For this review, take the finished solid that the model builds, in its own axes (mm). A direction names the side the tool comes from. Coordinates: 2 decimals unless noted, no trailing zeros. Write each loop counter-clockwise with the first axis right and the second up, starting at its lowest first coordinate (ties: lowest second). Pieces come first, ordered by that corner, then holes. Notation, with made-up numbers: (31.25, 74) - (49.25, 74) arc R23 ccw to (49.25, 100) - close; hole circle Ø3 at (58.25, -3.5). An arc over 180 degrees is marked (long way). Write each question's results on one line, items separated by ' | '.
from build123d import *

# Parameters (mm, degrees)
F0_W      = 140
F0_H      = 154
F1_DEPTH  = 54
F2_R      = 16
F3_DEPTH  = 140.001
F5_DEPTH  = 140.001
F6_W      = 25
F6_H      = 58
F7_DEPTH  = 46
F8_R      = 5
F9_ANGLE  = 270
F14_R     = 8
F15_DEPTH = 45
F16_R     = 5
F17_DEPTH = 120.001
F18_R     = 3
F19_DEPTH = 108.001


with BuildPart() as f1:
    # F0 (on Front) → F1 (new body, symmetric)
    with BuildSketch(Plane.XZ):
        with Locations((70, 0)):
            Rectangle(F0_W, F0_H)
    extrude(amount=F1_DEPTH, both=True)

    # F2 (on face) → F3 (cut, through all)
    with BuildSketch(Plane(origin=(0, 0, 0), x_dir=(0, -1, 0), z_dir=(-1, 0, 0))):
        with Locations((0, 48)):
            Circle(F2_R)
        with Locations((0, 3)):
            Circle(F2_R)
    extrude(amount=-F3_DEPTH, mode=Mode.SUBTRACT)

    # F4 (on face) → F5 (cut, through all)
    with BuildSketch(Plane(origin=(0, 0, 0), x_dir=(0, -1, 0), z_dir=(-1, 0, 0))):
        Polygon((-54, 77), (-54, 43), (-29, 43), (-29, 59.7311109304), (-11.6953058452, 77.0358050852), align=None)
        Polygon((54, 77), (11.6953058452, 77.0358050852), (29, 59.7311109304), (29, 43), (54, 43), align=None)
    extrude(amount=-F5_DEPTH, mode=Mode.SUBTRACT)

    # F6 (on face) → F7 (cut)
    with BuildSketch(Plane.XY.offset(77)):
        with Locations((127.5, 0)):
            Rectangle(F6_W, F6_H)
    extrude(amount=-F7_DEPTH, mode=Mode.SUBTRACT)

    # F8
    f8_edges = [f1.edges().sort_by_distance(p)[0] for p in [
        (127.5, -29, 31),
        (127.5, 29, 31),
    ]]
    fillet(f8_edges, radius=F8_R)


with BuildPart() as f1_1:
    # F9: moved
    add(f1.part.rotate(Axis((0, 0, -77), (0, 1, 0)), F9_ANGLE))


with BuildPart() as f1_2:
    # F11: moved
    add(f1_1.part.moved(Location((154, 0, 0))))


with BuildPart() as f1_3:
    # F13: moved
    add(f1_2.part.moved(Location((0, 0, 7))))

    # F14 (on face) → F15 (cut)
    with BuildSketch(Plane(origin=(0, 0, 0), x_dir=(0, -1, 0), z_dir=(-1, 0, 0))):
        with Locations((42, 38.6609129925)):
            Circle(F14_R)
        with Locations((-42, 38.6609129925)):
            Circle(F14_R)
        with Locations((42, -55.3390870075)):
            Circle(F14_R)
        with Locations((-42, -50)):
            Circle(F14_R)
    extrude(amount=-F15_DEPTH, mode=Mode.SUBTRACT)

    # F16 (on face) → F17 (cut, through all)
    with BuildSketch(Plane(origin=(34, 0, 0), x_dir=(0, -1, 0), z_dir=(-1, 0, 0))):
        with Locations((-42, -50)):
            Circle(F16_R)
        with Locations((-42, 38.6609129925)):
            Circle(F16_R)
        with Locations((42, 38.6609129925)):
            Circle(F16_R)
        with Locations((42, -55.3390870075)):
            Circle(F16_R)
    extrude(amount=-F17_DEPTH, mode=Mode.SUBTRACT)

    # F18 (on face) → F19 (cut, through all)
    with BuildSketch(Plane.XZ.offset(54)):
        with Locations((29, -55)):
            Circle(F18_R)
        with Locations((29, -31)):
            Circle(F18_R)
        with Locations((29, -7)):
            Circle(F18_R)
        with Locations((74, 55)):
            Circle(F18_R)
        with Locations((74, 31)):
            Circle(F18_R)
        with Locations((74, 7)):
            Circle(F18_R)
    extrude(amount=-F19_DEPTH, mode=Mode.SUBTRACT)


solid = f1_3.part
Q1. For faces 4 (the face through (26, -29, -13)), 5 (the face through (39.423, 48.349, 33.793)), 6 (the face through (26, 22, -31)), 7 (the face through (26, 29, -13)), 8 (the face through (37, -29, 57)), list the 3-axis set-ups (+Z, -Z, +X, -X, +Y, -Y) from which the entire face can be reached by the end or side of a thin tool; tool diameter is ignored.
Results found:
face 4: +Z, -Z, -X, -Y | face 5: -X | face 6: +Y, -Y | face 7: +Z, -Z, -X, +Y | face 8: +Z, -X
Q2. Mouldability with a two-part tool opening along X and no side actions: class faces 1 (the face through (26, 22, -7)), 2 (the face through (154, -1, -1)), 3 (the face through (98.74, -41.35, 43.62)) as pulls with the +X half, pulls with the -X half, needs draft (parallel to the pull), parting line crosses it, or undercut.
Results found:
face 1: undercut | face 2: pulls with the +X half | face 3: needs draft
Q3. Wall thickness on line 1 along Y through (x, z) = (119.5, 38); line 2 along X through (y, z) = (0, -42); line 3 along Z through (x, y) = (74, -36): over which ranges is each line inside the solid? List them lowest first. Write a range as from..to.
Results found:
line 1: -54..-46.96, -37.04..37.04, 46.96..54 | line 2: 0..13, 45..58, 90..154 | line 3: -70..4, 10..28, 34..52, 58..70
Q4. Take a section at C-C on y = -42. State the section outline as (x, z) points, plus the area to 3 significant figures.
Results found:
outline: (34, -70) - (154, -70) - (154, -60.34) - (45, -60.34) - (45, -63.34) - (34, -63.34) - close; (34, -47.34) - (45, -47.34) - (45, -50.34) - (154, -50.34) - (154, 33.66) - (75.39, 33.66) arc R3 cw (long way) to (72.61, 33.66) - (45, 33.66) - (45, 30.66) - (34, 30.66) - close; (34, 46.66) - (45, 46.66) - (45, 43.66) - (154, 43.66) - (154, 70) - (34, 70) - close; hole circle Ø6 at (74, 7); hole circle Ø6 at (74, 55) | area: 14,200 mm2
Q5. Take a section at D-D on z = -31. State the section outline as (x, y) points.
Results found:
outline: (0, -11.73) - (17.27, -29) - (26, -29) - (26, -15.72) arc R16 cw to (26, 15.72) - (26, 29) - (17.27, 29) - (0, 11.73) - close; (32, -29) - (34, -29) - (34, -54) - (154, -54) - (154, 54) - (34, 54) - (34, 29) - (32, 29) - (32, 15.72) arc R16 cw to (32, -15.72) - close; hole circle Ø32 at (74, 0)
Q6. Take a section at A-A on z = 7. State the section outline as (x, y) points, plus the area to 3 significant figures.
Results found:
outline: (0, -11.73) - (17.27, -29) - (34, -29) - (34, -54) - (71, -54) - (71, -15.72) arc R16 cw to (71, 15.72) - (71, 54) - (34, 54) - (34, 29) - (17.27, 29) - (0, 11.73) - close; (77, -54) - (154, -54) - (154, 54) - (77, 54) - (77, 15.72) arc R16 cw to (77, -15.72) - close; hole circle Ø32 at (29, 0) | area: 12,600 mm2
Q7. For pin 1 (8 mm diameter, centred on y = 38.5, z = 35.5, fed in from -X); pin 2 (5 mm diameter, centred on x = 28, z = 4, fed in from -Y); pin 3 (5 mm diameter, centred on x = 24.5, z = -36, fed in from +Y), all flat-tipped, find the tip position at first contact; note any pin that passes through.
Results found:
pin 1: x = 34 | pin 2: y = -29 | pin 3: y = 29
Q8. Take a section at B-B on z = 55. State the section outline as (x, y) points.
Results found:
outline: (34, -54) - (71, -54) - (71, -15.72) arc R16 cw to (71, 15.72) - (71, 54) - (34, 54) - (34, 29) - (41, 29) arc R5 cw to (46, 24) - (46, -24) arc R5 cw to (41, -29) - (34, -29) - close; (77, -54) - (154, -54) - (154, 54) - (77, 54) - (77, 15.72) arc R16 cw to (77, -15.72) - close
